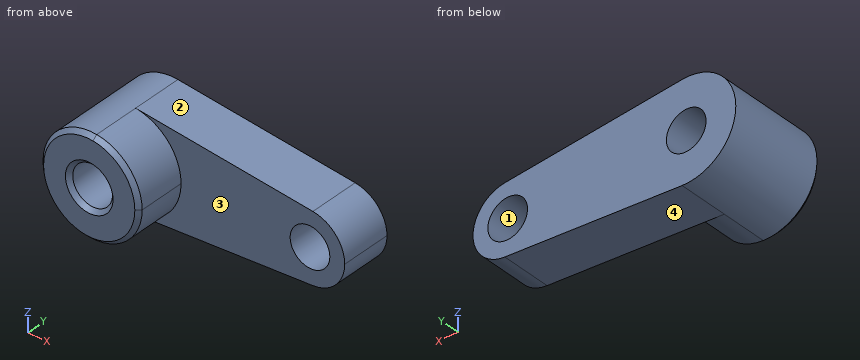
```python
from build123d import *

# Parameters (mm, degrees)
F0_R     = 10
F1_DEPTH = 25
F2_DEPTH = 50
F3_SIZE  = 2


with BuildPart() as f1:
    # F0 (on Front) → F1 (new body)
    with BuildSketch(Plane.XZ):
        with BuildLine():
            ThreePointArc((2.083333, -24.913043), (18.399502, -16.92508), (25, 0))
            ThreePointArc((25, 0), (18.399502, 16.92508), (2.083333, 24.913043))
            ThreePointArc((2.083333, 24.913043), (-25, 0), (2.083333, -24.913043))
        make_face()
        Circle(F0_R, mode=Mode.SUBTRACT)
        with BuildLine():
            ThreePointArc((2.083333, 24.913043), (18.399502, 16.92508), (25, 0))
            ThreePointArc((25, 0), (18.399502, -16.92508), (2.083333, -24.913043))
            Line((2.083333, -24.913043), (91.458333, -17.43913))
            ThreePointArc((91.458333, -17.43913), (72.5, 0), (91.458333, 17.43913))
            Line((91.458333, 17.43913), (2.083333, 24.913043))
        make_face()
        with BuildLine():
            ThreePointArc((107.5, 0), (102.879651, 11.847556), (91.458333, 17.43913))
            ThreePointArc((91.458333, 17.43913), (72.5, 0), (91.458333, -17.43913))
            ThreePointArc((91.458333, -17.43913), (102.879651, -11.847556), (107.5, 0))
        make_face()
        with Locations((90, 0)):
            Circle(F0_R, mode=Mode.SUBTRACT)
    extrude(amount=F1_DEPTH)

    # F0 (on Front) → F2 (join)
    with BuildSketch(Plane.XZ):
        with BuildLine():
            ThreePointArc((2.083333, -24.913043), (18.399502, -16.92508), (25, 0))
            ThreePointArc((25, 0), (18.399502, 16.92508), (2.083333, 24.913043))
            ThreePointArc((2.083333, 24.913043), (-25, 0), (2.083333, -24.913043))
        make_face()
        Circle(F0_R, mode=Mode.SUBTRACT)
    extrude(amount=F2_DEPTH)

    # F3
    f3_edges = [f1.edges().sort_by_distance(p)[0] for p in [
        (-2.083333, -50, 24.913043),
        (-10, -50, 0),
    ]]
    chamfer(f3_edges, length=F3_SIZE)


solid = f1.part
```
Geometry: final body of the model. Coordinates: model frame, mm. Face numbers are marked on the shaded views. Round coordinates to 2 decimals unless told otherwise and drop trailing zeros. Write each loop counter-clockwise with the first axis right and the second up, starting at its lowest first coordinate (ties: lowest second). Pieces come first, ordered by that corner, then holes.
Item 1: Material intervals for L1, parallel to Z at x = 0, y = -32; L2, parallel to Z at x = 86, y = -15.5; L3, parallel to Y at x = 35, z = -2, sorted ascending.
Item 2: Pin query (flat end, axial travel): P1, Ø8, axis at x = 12.5, y = -25.5, coming from the +Z side; P2, Ø6, axis at y = -18.5, z = -6.5, coming from the +X side; P3, Ø15, axis at x = 47, z = 12, coming from the -Y side. Return the tip coordinate at first contact, or that it passes through.
Item 3: Section query B-B (x = 90). Return loops of the section in (y, z).
Item 4: Section query D-D (x = 29.5). Return loops of the section in (y, z), plus the area to 3 significant figures.
Item 5: Section query A-A (y = -5.5). Return loops of the section in (x, z).
Item 6: Section query C-C (z = 4). Give the number of separate pieces and of enclosed holes in the cut face, plus the area to 3 significant figures.
Item 7: Mould query, pull axis Z, two halves, no side actions, for the marked faces 1, 2, 3 and 4. Classes: +Z half, -Z half, draft (parallel to the pull), parting line (faces both ways), or undercut.
Completed:
1. L1: z = -25 to -10, 10 to 25
1. L2: z = -17.9 to -9.17, 9.17 to 17.9
1. L3: y = -25 to 0
2. P1: stops at z = 24.37
2. P2: stops at x = 107.15
2. P3: stops at y = -25
3. outline: (-25, -17.56) - (0, -17.56) - (0, -10) - (-25, -10) - close; (-25, 10) - (0, 10) - (0, 17.56) - (-25, 17.56) - close
4. outline: (-25, -22.62) - (0, -22.62) - (0, 22.62) - (-25, 22.62) - close
4. area: 1,130 mm2
5. outline: (2.08, -24.91) - (91.46, -17.44) arc R17.5 ccw to (91.46, 17.44) - (2.08, 24.91) arc R25 ccw (long way) to start; hole circle Ø20 at (0, 0); hole circle Ø20 at (90, 0)
6. separate pieces: 3
6. enclosed holes: 0
6. area: 3,140 mm2
7. face 1: undercut
7. face 2: +Z half
7. face 3: draft
7. face 4: -Z half
